Geometry check sheet. Reference: the model listing, model coordinates, mm. A direction names the side the tool comes from. Give positions to 0.01 mm unless a question says otherwise; leave off trailing zeros. Write each loop counter-clockwise with the first axis right and the second up, starting at its lowest first coordinate (ties: lowest second). Pieces come first, ordered by that corner, then holes. Notation, with made-up numbers: (73.25, 18) -> (129.25, 18) arc R16 ccw to (129.25, 40) -> close; hole circle Ø9 at (27.5, 66). An arc over 180 degrees is marked (long way). One line per item, written item: value.
from build123d import *

# Parameters (mm, degrees)
BOSS_EXTRUDE1_DEPTH = 5.08
SKETCH2_R           = 27.051
CUT_EXTRUDE1_DEPTH  = 69.29129044


with BuildPart() as part:
    # Sketch1 → Boss-Extrude1 (new body)
    with BuildSketch(Plane(origin=(0, 0, 0), x_dir=(1, 0, 0), z_dir=(0, 1, 0))):
        with BuildLine():
            ThreePointArc((34.142692849, -3.175), (34.29, 0), (34.142692849, 3.175))
            Line((34.142692849, 3.175), (48.155445954, 3.175))
            ThreePointArc((48.155445954, 3.175), (34.12497326, 34.12497326), (3.175, 48.155445954))
            Line((3.175, 48.155445954), (3.175, 34.142692849))
            ThreePointArc((3.175, 34.142692849), (0, 34.29), (-3.175, 34.142692849))
            Line((-3.175, 34.142692849), (-3.175, 48.155445954))
            ThreePointArc((-3.175, 48.155445954), (-34.12497326, 34.12497326), (-48.155445954, 3.175))
            Line((-48.155445954, 3.175), (-34.142692849, 3.175))
            ThreePointArc((-34.142692849, 3.175), (-34.29, 0), (-34.142692849, -3.175))
            Line((-34.142692849, -3.175), (-48.155445954, -3.175))
            ThreePointArc((-48.155445954, -3.175), (-34.12497326, -34.12497326), (-3.175, -48.155445954))
            Line((-3.175, -48.155445954), (-3.175, -34.142692849))
            ThreePointArc((-3.175, -34.142692849), (0, -34.29), (3.175, -34.142692849))
            Line((3.175, -34.142692849), (3.175, -48.155445954))
            ThreePointArc((3.175, -48.155445954), (34.12497326, -34.12497326), (48.155445954, -3.175))
            Line((48.155445954, -3.175), (34.142692849, -3.175))
        make_face()
    extrude(amount=BOSS_EXTRUDE1_DEPTH)

    # Sketch2 → Cut-Extrude1 (cut, through all)
    with BuildSketch(Plane(origin=(0, 5.08, 0), x_dir=(1, 0, 0), z_dir=(0, 1, 0))):
        with Locations(Location((0, 0, 0), (0, 0, 270))):
            Circle(SKETCH2_R)
    extrude(amount=-CUT_EXTRUDE1_DEPTH, mode=Mode.SUBTRACT)


solid = part.part
1) Sectioned sample at D-D on x = -31. Record the cut outline in (y, z), plus the area to 3 significant figures.
Verdict:
outline: (0, -36.99) -> (5.08, -36.99) -> (5.08, 36.99) -> (0, 36.99) -> close
area: 376 mm^2
2) Tool access check on faces 1 (the flat face through (-3.175, 3, 41)), 2 (the flat face through (3.175, 3, -41)), 3 (the flat face through (-41, 3, 3.175)). Record the directions out of +Z, -Z, +X, -X, +Y, -Y that give a thin tool (end or side, any length) a straight path to the whole face; none if there is none.
Verdict:
face 1: +Z, +Y, -Y
face 2: -Z, +Y, -Y
face 3: -X, +Y, -Y
3) Scan lines: probe 1 along X at (y, z) = (2.7, 0); probe 2 along X at (y, z) = (4.4, -4.5); probe 3 along Z at (x, y) = (-39, 3) (3 decimals). Record each from-to range of solid material in increasing order.
Verdict:
probe 1: -34.29 to -27.05, 27.05 to 34.29
probe 2: -48.05 to -26.67, 26.67 to 48.05
probe 3: -28.426 to -3.175, 3.175 to 28.426
4) Sectioned sample at B-B on x = 0. Record the cut outline in (y, z).
Verdict:
outline: (0, -34.29) -> (5.08, -34.29) -> (5.08, -27.05) -> (0, -27.05) -> close; (0, 27.05) -> (5.08, 27.05) -> (5.08, 34.29) -> (0, 34.29) -> close
5) Depth check by flat-ended pin: pin 1 Ø2.5 at (y, z) = (3.5, 38.5) entering from -X; pin 2 Ø1 at (y, z) = (1.5, 26) entering from -X; pin 3 Ø1.5 at (y, z) = (2, 24) entering from +X. Enter the tip coordinate at first touch or a pass-through.
Verdict:
pin 1: x = -30.68
pin 2: x = -40.97
pin 3: x = 42.29
6) Sectioned sample at C-C on y = 3.7. Record the cut outline in (x, z) (3 decimals).
Verdict:
outline: (-48.155, -3.175) arc R48.26 ccw to (-3.175, -48.155) -> (-3.175, -34.143) arc R34.29 ccw to (3.175, -34.143) -> (3.175, -48.155) arc R48.26 ccw to (48.155, -3.175) -> (34.143, -3.175) arc R34.29 ccw to (34.143, 3.175) -> (48.155, 3.175) arc R48.26 ccw to (3.175, 48.155) -> (3.175, 34.143) arc R34.29 ccw to (-3.175, 34.143) -> (-3.175, 48.155) arc R48.26 ccw to (-48.155, 3.175) -> (-34.143, 3.175) arc R34.29 ccw to (-34.143, -3.175) -> close; hole circle Ø54.102 at (0, 0)
7) Sectioned sample at A-A on z = 0. Record the cut outline in (x, y), plus the area to 3 significant figures.
Verdict:
outline: (-34.29, 0) -> (-27.05, 0) -> (-27.05, 5.08) -> (-34.29, 5.08) -> close; (27.05, 0) -> (34.29, 0) -> (34.29, 5.08) -> (27.05, 5.08) -> close
area: 73.5 mm^2
8) Mould release check, pull along X, two halves, no side actions. Record for faces 4 (the cylindrical face through (34.29, 2.5, 0.04)), 5 (the flat face through (-41, 3, -3.175)), 6 (the flat face through (-3.175, 3, -41)), 7 (the cylindrical face through (-34.29, 2.5, -0.04)): released by +X, released by -X, zero draft, split by the parting line, or undercut.
Verdict:
face 4: released by +X
face 5: zero draft
face 6: undercut
face 7: released by -X
